```python
from build123d import *

# Parameters (mm, degrees)
F1_DEPTH = 63.5
F2_DEPTH = 25.4
F3_DEPTH = 12.7


with BuildPart() as f1:
    # F0 (on Front) → F1 (new body, symmetric)
    with BuildSketch(Plane.XZ):
        Polygon((-57.6780065894, 19.0542247146), (-57.6780065894, -19.0542247146), (57.6780065894, -19.0542247146), (57.6780065894, 19.0542247146), (25.1660067588, 19.0542247146), align=None)
    extrude(amount=F1_DEPTH, both=True)

    # F0 (on Front) → F2 (join, symmetric)
    with BuildSketch(Plane.XZ):
        with BuildLine():
            Line((170.935690403, 106.350377202), (97.6905226707, 106.350377202))
            add(Edge.make_bspline(
                [(97.6905226707, 106.350377202), (126.9282830626, 105.5487369377), (148.9319867328, 82.6442750732), (170.935690403, 59.7398132086)],
                knots=[0.5889393883, 0.5889393883, 0.5889393883, 0.5889393883, 1, 1, 1, 1], degree=3))
            Line((170.935690403, 59.7398132086), (170.935690403, 106.350377202))
        make_face()
        with BuildLine():
            add(Edge.make_bspline(
                [(97.6905226707, 106.350377202), (126.9282830626, 105.5487369377), (148.9319867328, 82.6442750732), (170.935690403, 59.7398132086)],
                knots=[0.5889393883, 0.5889393883, 0.5889393883, 0.5889393883, 1, 1, 1, 1], degree=3))
            Line((97.6905226707, 106.350377202), (97.6905226707, 100.020242855))
            Line((97.6905226707, 100.020242855), (97.6905226707, 67.5082430243))
            Line((97.6905226707, 67.5082430243), (97.6905226707, 59.7398132086))
            Line((97.6905226707, 59.7398132086), (170.935690403, 59.7398132086))
        make_face()
        with BuildLine():
            Line((25.1660067588, 19.0542247146), (57.6780065894, 19.0542247146))
            Line((57.6780065894, 19.0542247146), (57.6780065894, 44.2029610276))
            ThreePointArc((57.6780065894, 44.2029610276), (66.5609775012, 62.7717505439), (86.5927711129, 67.5082430243))
            Line((86.5927711129, 67.5082430243), (97.6905226707, 67.5082430243))
            Line((97.6905226707, 67.5082430243), (97.6905226707, 100.020242855))
            Line((97.6905226707, 100.020242855), (89.3401460729, 100.020242855))
            ThreePointArc((89.3401460729, 100.020242855), (44.5390942152, 86.7290974242), (25.1660067588, 44.2029610276))
            Line((25.1660067588, 44.2029610276), (25.1660067588, 19.0542247146))
        make_face()
    extrude(amount=F2_DEPTH, both=True)

    # F0 (on Front) → F3 (join)
    with BuildSketch(Plane.XZ):
        with BuildLine():
            add(Edge.make_bspline(
                [(-57.6780065894, 19.0542247146), (-0.9386686045, 63.2765684914), (55.8006693804, 107.4989122681), (97.6905226707, 106.350377202)],
                knots=[0, 0, 0, 0, 0.5889393883, 0.5889393883, 0.5889393883, 0.5889393883], degree=3))
            Line((-57.6780065894, 19.0542247146), (25.1660067588, 19.0542247146))
            Line((25.1660067588, 19.0542247146), (25.1660067588, 44.2029610276))
            ThreePointArc((25.1660067588, 44.2029610276), (44.5390942152, 86.7290974242), (89.3401460729, 100.020242855))
            Line((89.3401460729, 100.020242855), (97.6905226707, 100.020242855))
            Line((97.6905226707, 100.020242855), (97.6905226707, 106.350377202))
        make_face()
    extrude(amount=F3_DEPTH)


solid = f1.part
```
Source: CAD feature listing. Evaluate the final solid. Frame: model axes, mm. A direction names the side the tool comes from. Coordinates: 2 decimals unless noted, no trailing zeros. Loops run counter-clockwise (first coordinate to the right, second up) from the corner with the lowest first, then second, coordinate; pieces in that order, holes last. Notation, with made-up numbers: M 38.5,-2.75 L 76.5,-2.75 A25 cw 76.5,10.25 Z; hole C 9,2 d1. An arc over 180 degrees is marked long. Use CSV: the item, a comma, the result in double quotes.
(1) Line query: line 1 (X direction, y = 38, z = 12.5); line 2 (Y direction, x = 12.5, z = 31); line 3 (X direction, y = 7, z = 21). Output: solid intervals per line, ascending. Write a range as [from, to].
Answers follow:
line 1,"[-57.68, 57.68]"
line 2,"[-12.7, 0]"
line 3,"[25.17, 57.68]"
(2) Cut plane C-C on z = 4. Return loops of the section in (x, y), and give its area (3 significant figures).
Answers follow:
outline,"M -57.68,-63.5 L 57.68,-63.5 L 57.68,63.5 L -57.68,63.5 Z"
area,"14,700 mm²"
(3) Contact query for flat-ended pins moving along their axis: pin 1 (3 mm diameter, centred on y = 0, z = 17.5, fed in from +X); pin 2 (6.5 mm diameter, centred on x = 92, y = 13, fed in from +Z); pin 3 (12 mm diameter, centred on x = 90, y = 12.5, fed in from -Z). Output: stop coordinate, or through.
Answers follow:
pin 1,"x = 57.68"
pin 2,"z = 100.1"
pin 3,"z = 67.51"
(4) Cut plane B-B on x = 140. Return loops of the section in (y, z).
Answers follow:
outline,"M -25.4,59.74 L 25.4,59.74 L 25.4,106.35 L -25.4,106.35 Z"
(5) Reachability of faces 1 (the face through (97.691, 0, 64)), 2 (the face through (97, -25.4, 73)), 3 (the face through (25.166, 13, 32)), 4 (the face through (57.678, -1, 5)), 5 (the face through (94, -19, 100.02)) from +Z, -Z, +X, -X, +Y, -Y: full face, straight path, thin tool, end or side. Return the list, or none.
Answers follow:
face 1,"-Z, +Y, -Y"
face 2,"+Z, +X, -X, -Y"
face 3,"+Z, -X, +Y"
face 4,"-Z, +X, +Y, -Y"
face 5,"+Z, -Y"
(6) Cut plane A-A on y = 18. Return loops of the section in (x, z), and give its area (3 significant figures).
Answers follow:
outline,"M -57.68,-19.05 L 57.68,-19.05 L 57.68,44.2 A23.85 cw 86.59,67.51 L 97.69,67.51 L 97.69,59.74 L 170.94,59.74 L 170.94,106.35 L 97.69,106.35 L 97.69,100.02 L 89.34,100.02 A56.36 ccw 25.17,44.2 L 25.17,19.05 L -57.68,19.05 Z"
area,"11,200 mm²"
